```python
from build123d import *

# Parameters (mm, degrees)
SKETCH1_W           = 26
SKETCH1_H           = 5
BOSS_EXTRUDE1_DEPTH = 5
FILLET1_R           = 50
SKETCH1_5_W         = 26
SKETCH1_5_H         = 5
BOSS_EXTRUDE2_DEPTH = 20


with BuildPart() as part:
    # Sketch1 → Boss-Extrude1 (new body)
    with BuildSketch(Plane.XY):
        Polygon((9.235124147, 168.867198813), (-470.476307556, -108.094325414), (9.235124147, -385.055849641), align=None)
        with Locations((-7.764875853, -285.594325414)):
            Rectangle(SKETCH1_W, SKETCH1_H, mode=Mode.SUBTRACT)
        Polygon((-64.066146043, -308.094325414), (-59.736019024, -310.594325414), (-72.736019024, -333.110985912), (-77.066146043, -330.610985912), align=None, mode=Mode.SUBTRACT)
        Polygon((-371.505164386, -130.594325414), (-367.175037367, -133.094325414), (-380.175037367, -155.610985912), (-384.505164386, -153.110985912), align=None, mode=Mode.SUBTRACT)
        Polygon((-367.175037367, -83.094325414), (-371.505164386, -85.594325414), (-384.505164386, -63.077664915), (-380.175037367, -60.577664915), align=None, mode=Mode.SUBTRACT)
        Polygon((-59.736019024, 94.405674586), (-64.066146043, 91.905674586), (-77.066146043, 114.422335085), (-72.736019024, 116.922335085), align=None, mode=Mode.SUBTRACT)
        with Locations((-7.764875853, 69.405674586)):
            Rectangle(SKETCH1_W, SKETCH1_H, mode=Mode.SUBTRACT)
    extrude(amount=BOSS_EXTRUDE1_DEPTH)

    # Fillet1
    fillet1_edges = [part.edges().sort_by_distance(p)[0] for p in [
        (-470.476307556, -108.094325414, 2.5),
        (9.235124147, 168.867198813, 2.5),
        (9.235124147, -385.055849641, 2.5),
    ]]
    fillet(fillet1_edges, radius=FILLET1_R)

    # Sketch1<5> → Boss-Extrude2 (add)
    with BuildSketch(Plane.XY):
        with Locations((-7.764875853, 69.405674586)):
            Rectangle(SKETCH1_5_W, SKETCH1_5_H)
        Polygon((-64.066146043, 91.905674586), (-59.736019024, 94.405674586), (-72.736019024, 116.922335085), (-77.066146043, 114.422335085), align=None)
        Polygon((-371.505164386, -85.594325414), (-367.175037367, -83.094325414), (-380.175037367, -60.577664915), (-384.505164386, -63.077664915), align=None)
        Polygon((-380.175037367, -155.610985912), (-367.175037367, -133.094325414), (-371.505164386, -130.594325414), (-384.505164386, -153.110985912), align=None)
        Polygon((-72.736019024, -333.110985912), (-59.736019024, -310.594325414), (-64.066146043, -308.094325414), (-77.066146043, -330.610985912), align=None)
        with Locations((-7.764875853, -285.594325414)):
            Rectangle(SKETCH1_5_W, SKETCH1_5_H)
    extrude(amount=BOSS_EXTRUDE2_DEPTH)


solid = part.part
```
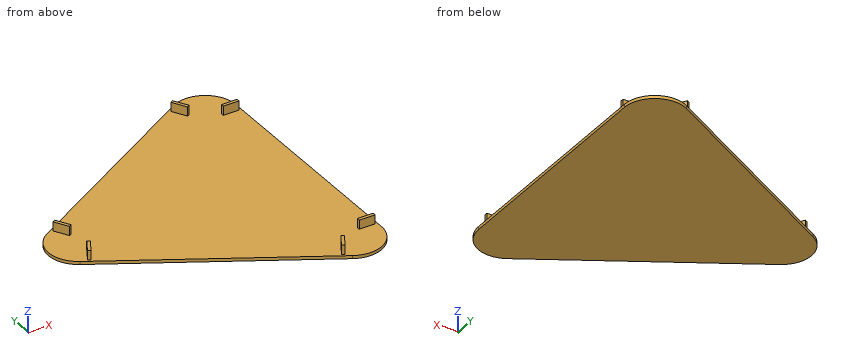
The model under review builds one solid part; all positions refer to its coordinate system, in mm. Round coordinates to 2 decimals unless told otherwise and drop trailing zeros. Loops run counter-clockwise (first coordinate to the right, second up) from the corner with the lowest first, then second, coordinate; pieces in that order, holes last. Notation, with made-up numbers: M -2,37 L 25,37 A22 cw 25,66 Z; hole C 2.5,82.25 d10. An arc over 180 degrees is marked long. Write item = value, one per line.
Item 1: Take a section at C-C on x = -233.5. Write out the cut boundary in (y, z), then the cut area to 3 significant figures.
Return value:
outline = M -244.91,0 L 28.72,0 L 28.72,5 L -244.91,5 Z
area = 1,370 mm2
Item 2: Take a section at A-A on z = 8.75. Write out the cut boundary in (x, y).
Return value:
outline = M -384.51,-153.11 L -380.18,-155.61 L -367.18,-133.09 L -371.51,-130.59 Z; M -384.51,-63.08 L -371.51,-85.59 L -367.18,-83.09 L -380.18,-60.58 Z; M -77.07,-330.61 L -72.74,-333.11 L -59.74,-310.59 L -64.07,-308.09 Z; M -77.07,114.42 L -64.07,91.91 L -59.74,94.41 L -72.74,116.92 Z; M -20.76,-288.09 L 5.24,-288.09 L 5.24,-283.09 L -20.76,-283.09 Z; M -20.76,66.91 L 5.24,66.91 L 5.24,71.91 L -20.76,71.91 Z
Item 3: Insertion check: P1, Ø1.5, axis at y = -286.5, z = 15.5, coming from the +X side; P2, Ø2.5, axis at y = 69.5, z = 14, coming from the -X side; P3, Ø10, axis at x = -125.5, z = 4.5, coming from the -Y side. Each pin has a flat end and moves straight along its axis. Give the tip position at first contact, or say it passes through.
Return value:
P1 = 5.24
P2 = -20.76
P3 = -310.15
Item 4: Take a section at D-D on y = -8.5. Write out the cut boundary in (x, z), then the cut area to 3 significant figures.
Return value:
outline = M -297.97,0 L 9.24,0 L 9.24,5 L -297.97,5 Z
area = 1,540 mm2
Item 5: For line 1 (Z direction, x = -87, y = -58); line 2 (X direction, y = -81.5, z = 8.5); line 3 (X direction, y = -188.5, z = 1.25), list the stretches that pass through material, from the lowest coordinate up. Write a range as [from, to].
Return value:
line_1 = [0, 5]
line_2 = [-373.87, -368.1]
line_3 = [-331.21, 9.24]
Item 6: Take a section at B-B on y = 100.5. Write out the cut boundary in (x, z), then the cut area to 3 significant figures.
Return value:
outline = M -109.18,0 L 5.79,0 L 5.79,5 L -63.25,5 L -63.25,20 L -69.03,20 L -69.03,5 L -109.18,5 Z
area = 661 mm2
